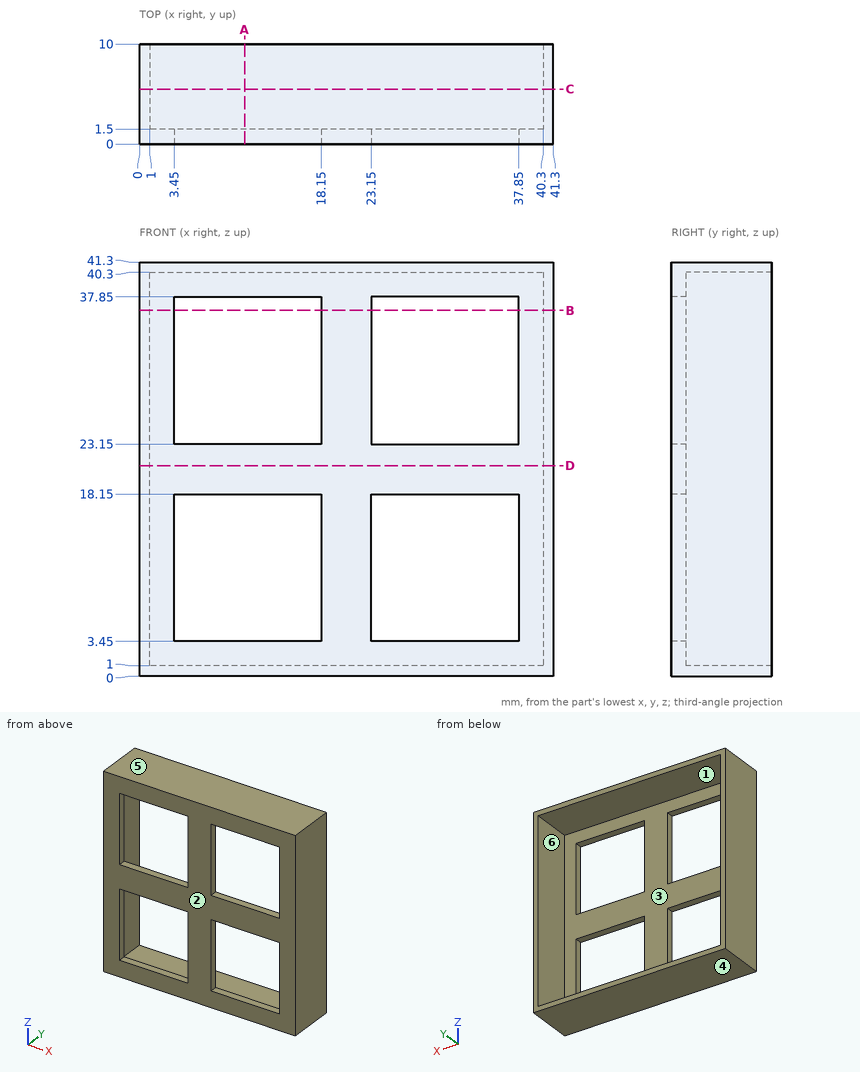
The figure shows three views and two pictorial views of one solid part (mm, origin at its lowest corner). Answer the questions. A direction names the side the tool comes from. Round coordinates to 2 decimals unless told otherwise and drop trailing zeros. Write each loop counter-clockwise with the first axis right and the second up, starting at its lowest first coordinate (ties: lowest second). Pieces come first, ordered by that corner, then holes. Notation, with made-up numbers: (-5.75, -29.75) -> (46.25, -29.75) arc R36 cw to (46.25, 5.25) -> close; hole circle Ø7 at (2, 78). An arc over 180 degrees is marked (long way). Answer as a JSON object with one key per item and string values. Group by question number.
Q1. Section C-C (y = 5.5) is taken. Write down the section's boundary in (x, z), plus the area to 3 significant figures.
Q2. Section B-B (z = 36.5) is taken. Write down the section's boundary in (x, y).
Q3. Determine the mould class of the marked faces 3, 4, 5 and 6 for opening direction Z: pulls with the +Z half, pulls with the -Z half, needs draft (parallel to the pull), parting line crosses it, or undercut.
Q4. Section A-A (x = 10.5) is taken. Write down the section's boundary in (y, z), plus the area to 4 significant figures.
Q5. Section D-D (z = 21) is taken. Write down the section's boundary in (x, y), plus the area to 4 significant figures.
Q6. Each of these flat-tipped pins is pushed along its axis until it touches: pin 1 Ø1.2 at (y, z) = (1, 27.5) entering from -X; pin 2 Ø19.5 at (x, z) = (21.5, 19) entering from +Y. Where does it stop, or does it pass through?
Q7. Which of the six approach directions +Z, -Z, +X, -X, +Y, -Y give full straight-line access (tool end or side, diameter ignored) to the marked faces 1 and 2?
Q8. Straight lines are drawn through the part: line 1 along Z through (x, y) = (31, 0.75); line 2 along X through (y, z) = (7.25, 35). For each, find the intervals that lie inside material, in ascending order.
Check values:
{
 "1": {"outline": "(0, 0) -> (41.3, 0) -> (41.3, 41.3) -> (0, 41.3) -> close; hole (1, 1) -> (40.3, 1) -> (40.3, 40.3) -> (1, 40.3) -> close", "area": "161 mm^2"},
 "2": {"outline": "(0, 0) -> (3.45, 0) -> (3.45, 1.5) -> (1, 1.5) -> (1, 10) -> (0, 10) -> close; (18.15, 0) -> (23.15, 0) -> (23.15, 1.5) -> (18.15, 1.5) -> close; (37.85, 0) -> (41.3, 0) -> (41.3, 10) -> (40.3, 10) -> (40.3, 1.5) -> (37.85, 1.5) -> close"},
 "3": {"face 3": "undercut", "face 4": "pulls with the -Z half", "face 5": "pulls with the +Z half", "face 6": "undercut"},
 "4": {"outline": "(0, 0) -> (10, 0) -> (10, 1) -> (1.5, 1) -> (1.5, 3.45) -> (0, 3.45) -> close; (0, 18.15) -> (1.5, 18.15) -> (1.5, 23.15) -> (0, 23.15) -> close; (0, 37.85) -> (1.5, 37.85) -> (1.5, 40.3) -> (10, 40.3) -> (10, 41.3) -> (0, 41.3) -> close", "area": "34.85 mm^2"},
 "5": {"outline": "(0, 0) -> (41.3, 0) -> (41.3, 10) -> (40.3, 10) -> (40.3, 1.5) -> (1, 1.5) -> (1, 10) -> (0, 10) -> close", "area": "78.95 mm^2"},
 "6": {"pin 1": "x = 0", "pin 2": "y = 1.5"},
 "7": {"face 1": "+Y", "face 2": "+Z, -Z, +X, -X, -Y"},
 "8": {"line 1": "0 to 3.45, 18.15 to 23.15, 37.85 to 41.3", "line 2": "0 to 1, 40.3 to 41.3"}
}
